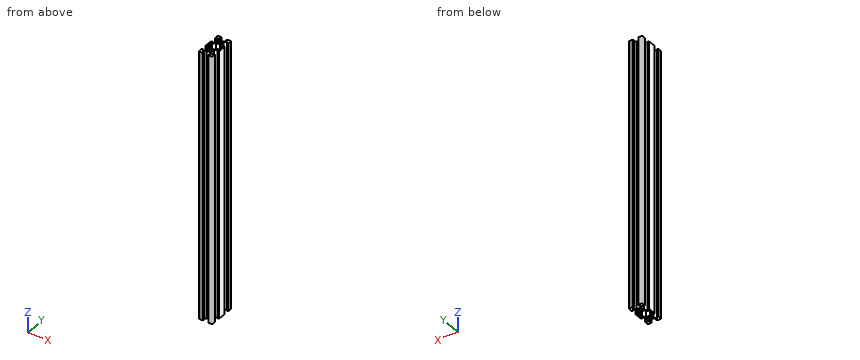
Autodesk Inventor part; units mm, degrees
ref_plane "Work Plane1" through (4.58, 10, 197.5) normal (0, 1, 0) x (1, 0, 0)
ref_plane "YZ Plane" through (0, 0, 0) normal (1, 0, 0) x (0, 1, 0)
ref_plane "XZ Plane" through (0, 0, 0) normal (0, 1, 0) x (-1, 0, 0)
sketch "Sketch1" plane through (0, 0, 0) normal (0, 0, 1) x (1, 0, 0)
  line L0 (0, 3.7) -> (-2.6393, 3.7)
  line L1 (-2.6393, 3.7) -> (-5.5, 6.5607)
  line L2 (-5.5, 6.5607) -> (-5.5, 8.2)
  line L3 (-5.5, 8.2) -> (-3.395, 8.2)
  line L4 (-3.395, 8.2) -> (-3.395, 10)
  line L5 (-3.395, 10) -> (-10, 10)
  line L6 (-10, 10) -> (-10, 3.395)
  line L7 (-10, 3.395) -> (-8.2, 3.395)
  line L8 (-8.2, 3.395) -> (-8.2, 5.5)
  line L9 (-8.2, 5.5) -> (-6.5607, 5.5)
  line L10 (-6.5607, 5.5) -> (-3.7, 2.6393)
  line L11 (-3.7, 2.6393) -> (-3.7, 0)
  line L12 (0, 0) -> (-10, 10) construction
  circle A0 centre (0, 0) radius 2.3
  line L13 (-22.6601, 0) -> (65.9605, 0)
  line L14 (-3.7, 0) -> (0, 0)
  line L15 (0, 0) -> (0, 3.7)
  line L16 (11.2521, 18.9743) -> (53.3004, 18.9743) construction
  line L17 (53.3004, 18.9743) -> (53.3004, -5.624) construction
  line L18 (53.3004, -5.624) -> (11.2521, -5.624) construction
  line L19 (11.2521, -5.624) -> (11.2521, 18.9743) construction
  point P0 (-2.3, 0)
  point P1 (0, 2.3)
  dimension "d0" = 1.5
  dimension "d6" = 6.3
  dimension "d9" = 4.6
  dimension "d18" = 135
  dimension "d22" = 20
  dimension "d34" = 11
  dimension "d35" = 6.79
  dimension "d36" = 1.8
extrude "Extrusion1" add sketch "Sketch1" along normal mid plane 395 contours L15 A0 L13 L11 L10 L9 L8 L7 L6 L5 L4 L3 L2 L1 L0
pattern_circular "Circular Pattern1" count 4 over 360 about axis through (0, 0, -10) along (0, 0, 1) of "Extrusion1"
chamfer "Chamfer1" distance 1.185 angle 45 8 edges at (-3.395, 10, 0) (3.395, 10, 0) (10, 3.395, 0) (10, -3.395, 0) (3.395, -10, 0) (-3.395, -10, 0) (-10, -3.395, 0) (-10, 3.395, 0)
ref_plane "Work Plane1" through (4.58, 10, 197.5) normal (0, 1, 0) x (1, 0, 0)
mirror "Mirror1" about plane through (4.58, 10, 197.5) normal (0, 1, 0)
sketch "Sketch2" plane through (0, 0, 197.5) normal (0, 0, 1) x (1, 0, 0)
  line L0 (-10, 4.58) -> (-10, 15.42)
  line L1 (-8.815, 3.395) -> (-10, 4.58)
  line L2 (-8.815, 3.395) -> (-8.2, 3.395)
  line L3 (-8.2, 3.395) -> (-8.2, 5.5)
  line L4 (-8.2, 5.5) -> (-6.5607, 5.5)
  line L5 (-6.5607, 5.5) -> (-3.7, 2.6393)
  line L6 (-3.7, -2.6393) -> (-6.5607, -5.5)
  line L7 (-6.5607, -5.5) -> (-8.2, -5.5)
  line L8 (-8.2, -5.5) -> (-8.2, -3.395)
  line L9 (-8.2, -3.395) -> (-8.815, -3.395)
  line L10 (-10, -4.58) -> (-8.815, -3.395)
  line L11 (-10, -4.58) -> (-10, -10)
  line L12 (-10, -10) -> (-4.58, -10)
  line L13 (-3.395, -8.815) -> (-4.58, -10)
  line L14 (-3.395, -8.815) -> (-3.395, -8.2)
  line L15 (-3.395, -8.2) -> (-5.5, -8.2)
  line L16 (-5.5, -8.2) -> (-5.5, -6.5607)
  line L17 (-5.5, -6.5607) -> (-2.6393, -3.7)
  line L18 (2.6393, -3.7) -> (5.5, -6.5607)
  line L19 (5.5, -6.5607) -> (5.5, -8.2)
  line L20 (5.5, -8.2) -> (3.395, -8.2)
  line L21 (3.395, -8.2) -> (3.395, -8.815)
  line L22 (4.58, -10) -> (3.395, -8.815)
  line L23 (4.58, -10) -> (10, -10)
  line L24 (10, -10) -> (10, -4.58)
  line L25 (8.815, -3.395) -> (10, -4.58)
  line L26 (8.815, -3.395) -> (8.2, -3.395)
  line L27 (8.2, -3.395) -> (8.2, -5.5)
  line L28 (8.2, -5.5) -> (6.5607, -5.5)
  line L29 (6.5607, -5.5) -> (3.7, -2.6393)
  line L30 (3.7, 2.6393) -> (6.5607, 5.5)
  line L31 (6.5607, 5.5) -> (8.2, 5.5)
  line L32 (8.2, 5.5) -> (8.2, 3.395)
  line L33 (8.2, 3.395) -> (8.815, 3.395)
  line L34 (10, 4.58) -> (8.815, 3.395)
  line L35 (10, 4.58) -> (10, 15.42)
  line L36 (10, 15.42) -> (8.815, 16.605)
  line L37 (8.2, 16.605) -> (8.815, 16.605)
  line L38 (8.2, 14.5) -> (8.2, 16.605)
  line L39 (6.5607, 14.5) -> (8.2, 14.5)
  line L40 (3.7, 17.3607) -> (6.5607, 14.5)
  line L41 (6.5607, 25.5) -> (3.7, 22.6393)
  line L42 (8.2, 25.5) -> (6.5607, 25.5)
  line L43 (8.2, 23.395) -> (8.2, 25.5)
  line L44 (8.815, 23.395) -> (8.2, 23.395)
  line L45 (8.815, 23.395) -> (10, 24.58)
  line L46 (10, 30) -> (10, 24.58)
  line L47 (4.58, 30) -> (10, 30)
  line L48 (4.58, 30) -> (3.395, 28.815)
  line L49 (3.395, 28.2) -> (3.395, 28.815)
  line L50 (5.5, 28.2) -> (3.395, 28.2)
  line L51 (5.5, 26.5607) -> (5.5, 28.2)
  line L52 (2.6393, 23.7) -> (5.5, 26.5607)
  line L53 (-5.5, 26.5607) -> (-2.6393, 23.7)
  line L54 (-5.5, 28.2) -> (-5.5, 26.5607)
  line L55 (-3.395, 28.2) -> (-5.5, 28.2)
  line L56 (-3.395, 28.815) -> (-3.395, 28.2)
  line L57 (-3.395, 28.815) -> (-4.58, 30)
  line L58 (-10, 30) -> (-4.58, 30)
  line L59 (-10, 24.58) -> (-10, 30)
  line L60 (-10, 24.58) -> (-8.815, 23.395)
  line L61 (-8.2, 23.395) -> (-8.815, 23.395)
  line L62 (-8.2, 25.5) -> (-8.2, 23.395)
  line L63 (-6.5607, 25.5) -> (-8.2, 25.5)
  line L64 (-3.7, 22.6393) -> (-6.5607, 25.5)
  line L65 (-6.5607, 14.5) -> (-3.7, 17.3607)
  line L66 (-8.2, 14.5) -> (-6.5607, 14.5)
  line L67 (-8.2, 16.605) -> (-8.2, 14.5)
  line L68 (-8.815, 16.605) -> (-8.2, 16.605)
  line L69 (-8.815, 16.605) -> (-10, 15.42)
  circle A0 centre (0, 20) radius 2.3
  line L70 (-4.58, 10) -> (-3.395, 11.185)
  line L71 (-3.395, 11.8) -> (-3.395, 11.185)
  line L72 (-5.5, 11.8) -> (-3.395, 11.8)
  line L73 (-5.5, 13.4393) -> (-5.5, 11.8)
  line L74 (-2.6393, 16.3) -> (-5.5, 13.4393)
  line L75 (5.5, 13.4393) -> (2.6393, 16.3)
  line L76 (5.5, 11.8) -> (5.5, 13.4393)
  line L77 (3.395, 11.8) -> (5.5, 11.8)
  line L78 (3.395, 11.185) -> (3.395, 11.8)
  line L79 (3.395, 11.185) -> (4.58, 10)
  line L80 (3.395, 8.815) -> (4.58, 10)
  line L81 (3.395, 8.815) -> (3.395, 8.2)
  line L82 (3.395, 8.2) -> (5.5, 8.2)
  line L83 (5.5, 8.2) -> (5.5, 6.5607)
  line L84 (5.5, 6.5607) -> (2.6393, 3.7)
  line L85 (-2.6393, 3.7) -> (-5.5, 6.5607)
  line L86 (-5.5, 6.5607) -> (-5.5, 8.2)
  line L87 (-5.5, 8.2) -> (-3.395, 8.2)
  line L88 (-3.395, 8.2) -> (-3.395, 8.815)
  line L89 (-4.58, 10) -> (-3.395, 8.815)
  circle A1 centre (0, 0) radius 2.3
  line L90 (-5.5, 8.2) -> (-5.5, 6.5607)
  line L91 (-5.5, 6.5607) -> (-6.2393, 7.3)
  line L92 (-5.5, 6.5607) -> (-2.6393, 3.7)
  line L93 (-6.2393, 7.3) -> (-8.2, 7.3)
  line L94 (-8.2, 7.3) -> (-8.2, 12.7)
  line L95 (-8.2, 12.7) -> (-6.2393, 12.7)
  line L96 (-6.2393, 12.7) -> (-5.5, 13.4393)
  line L97 (-2.6393, 16.3) -> (-5.5, 13.4393)
  line L98 (-8.2, 16.605) -> (-8.2, 14.5)
  line L99 (-3.7, 2.6393) -> (-3.7, -2.6393)
  line L100 (-2.6393, -3.7) -> (2.6393, -3.7)
  line L101 (3.7, -2.6393) -> (3.7, 2.6393)
  line L102 (3.7, 22.6393) -> (3.7, 17.3607)
  line L103 (-2.6393, 23.7) -> (2.6393, 23.7)
  line L104 (-3.7, 17.3607) -> (-3.7, 22.6393)
  line L105 (2.6393, 16.3) -> (-2.6393, 16.3)
  line L106 (2.6393, 3.7) -> (-2.6393, 3.7)
  dimension "d42" = 1.8
extrude "Extrusion2" cut sketch "Sketch2" against normal through all contours L89 L88 L87 L86 L91 L93 L94 L95 L96 L73 L72 L71 L70
fillet "Fillet2" radius 1.5 4 edges at (-10, 30, 0) (10, 30, 0) (10, -10, 0) (-10, -10, 0)
mirror "Mirror2" about plane through (0, 0, 0) normal (1, 0, 0) of "Extrusion2"
equation "\"d24\" = WorkspaceLength"
equation "\"GridProcutClearance\" = 3"
equation "\"GridBorderThickness\" = 5"
equation "\"GridBorderFillets\" = 7"
equation "\"GridTotalSize\" = 63"
equation "\"BaseTotalWidth\" = 412"
equation "\"BaseTotalLength\" = 624"
equation "\"DistanceBetweenGrid\" = 5"
equation "\"WorkspaceLength\" = 395"
equation "\"WorkspaceWidth\" = 332"
equation "\"AxesBaseFillet\" = 15"
equation "\"Zaxis\" = 127"
properties part number "2040aluminum_extrusion_black" material "Aluminum 6061"
Geometry: final body of the model. Coordinates: model frame, mm. Round coordinates to 2 decimals unless told otherwise and drop trailing zeros. Use CSV: the item, a comma, the result in double quotes. Start each with the question number.
Q1. Section A-A (z = -37). Give the number of separate pieces and of enclosed holes in the cut face, plus the area to 3 significant figures.
Q2. Line query: L1, parallel to Y at x = 8.25, z = 141.5 (3 decimals); L2, parallel to Y at x = 0, z = -41.5; L3, parallel to Y at x = -7.5, z = 79.5. Output: solid intervals per line, ascending.
Q3. First-contact query: pin 1 Ø3 at (x, y) = (0, 0) entering from +Z; pin 2 Ø4 at (x, z) = (0, -92.5) entering from +Y; pin 3 Ø2 at (x, z) = (-2.5, -132) entering from +Y; pin 4 Ø1.5 at (y, z) = (17.5, 39.5) entering from -X. Flat tips, straight axial feed; report the tip coordinate or a pass-through.
Result sheet:
1,separate pieces,"1"
1,enclosed holes,"3"
1,area,"283 mm²"
2,L1,"-10 to -3.395, 3.395 to 16.605, 23.395 to 30"
2,L2,"-3.7 to -2.3, 2.3 to 3.7, 16.3 to 17.7, 22.3 to 23.7"
2,L3,"-10 to -5.5, 5.5 to 7.3, 12.7 to 14.5, 25.5 to 30"
3,pin 1,"through"
3,pin 2,"y = 23.7"
3,pin 3,"y = 28.92"
3,pin 4,"x = -4.31"
